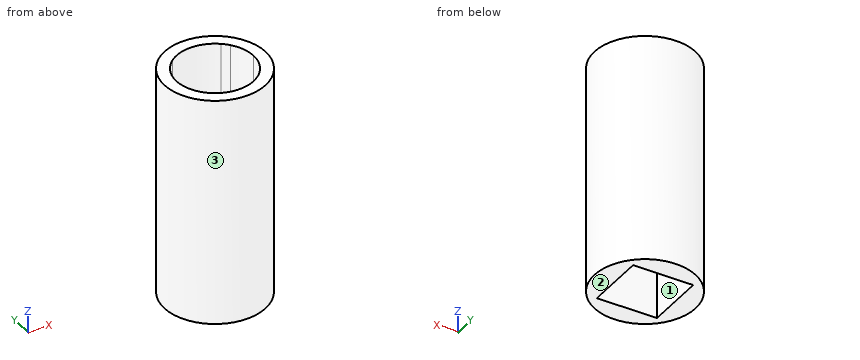
```python
from build123d import *

# Parameters (mm, degrees)
F0_R     = 21
F0_W     = 24.95
F0_H     = 24.95
F1_DEPTH = 45
F2_R     = 21
F3_DEPTH = 50
F4_DEPTH = 5


with BuildPart() as f1:
    # F0 (on Top) → F1 (new body)
    with BuildSketch(Plane.XY):
        Circle(F0_R)
        Rectangle(F0_W, F0_H, mode=Mode.SUBTRACT)
    extrude(amount=F1_DEPTH)

    # F2 (on face) → F3 (join)
    with BuildSketch(Plane.XY.offset(45)):
        Circle(F2_R)
        with BuildLine():
            ThreePointArc((12.475, 10.0585784284), (15.1114608824, 5.3333268229), (16.025, 0))
            ThreePointArc((16.025, 0), (15.1114608824, -5.3333268229), (12.475, -10.0585784284))
            Line((12.475, -10.0585784284), (12.475, -12.475))
            Line((12.475, -12.475), (10.0585784284, -12.475))
            ThreePointArc((10.0585784284, -12.475), (0, -16.025), (-10.0585784284, -12.475))
            Line((-10.0585784284, -12.475), (-12.475, -12.475))
            Line((-12.475, -12.475), (-12.475, -10.0585784284))
            ThreePointArc((-12.475, -10.0585784284), (-16.025, 0), (-12.475, 10.0585784284))
            Line((-12.475, 10.0585784284), (-12.475, 12.475))
            Line((-12.475, 12.475), (-10.0585784284, 12.475))
            ThreePointArc((-10.0585784284, 12.475), (0, 16.025), (10.0585784284, 12.475))
            Line((10.0585784284, 12.475), (12.475, 12.475))
            Line((12.475, 12.475), (12.475, 10.0585784284))
        make_face(mode=Mode.SUBTRACT)
        with BuildLine():
            ThreePointArc((10.0585784284, 12.475), (11.3313861685, 11.3313861685), (12.475, 10.0585784284))
            Line((12.475, 10.0585784284), (12.475, 12.475))
            Line((12.475, 12.475), (10.0585784284, 12.475))
        make_face()
        with BuildLine():
            Line((12.475, -12.475), (12.475, -10.0585784284))
            ThreePointArc((12.475, -10.0585784284), (11.3313861685, -11.3313861685), (10.0585784284, -12.475))
            Line((10.0585784284, -12.475), (12.475, -12.475))
        make_face()
        with BuildLine():
            ThreePointArc((-12.475, 10.0585784284), (-11.3313861685, 11.3313861685), (-10.0585784284, 12.475))
            Line((-10.0585784284, 12.475), (-12.475, 12.475))
            Line((-12.475, 12.475), (-12.475, 10.0585784284))
        make_face()
        with BuildLine():
            Line((-12.475, -12.475), (-10.0585784284, -12.475))
            ThreePointArc((-10.0585784284, -12.475), (-11.3313861685, -11.3313861685), (-12.475, -10.0585784284))
            Line((-12.475, -10.0585784284), (-12.475, -12.475))
        make_face()
    extrude(amount=F3_DEPTH)

    # F2 (on face) → F4 (join)
    with BuildSketch(Plane.XY.offset(45)):
        with BuildLine():
            Line((12.475, -10.0585784284), (12.475, 10.0585784284))
            ThreePointArc((12.475, 10.0585784284), (11.3313861685, 11.3313861685), (10.0585784284, 12.475))
            Line((10.0585784284, 12.475), (-10.0585784284, 12.475))
            ThreePointArc((-10.0585784284, 12.475), (-11.3313861685, 11.3313861685), (-12.475, 10.0585784284))
            Line((-12.475, 10.0585784284), (-12.475, -10.0585784284))
            ThreePointArc((-12.475, -10.0585784284), (-11.3313861685, -11.3313861685), (-10.0585784284, -12.475))
            Line((-10.0585784284, -12.475), (10.0585784284, -12.475))
            ThreePointArc((10.0585784284, -12.475), (11.3313861685, -11.3313861685), (12.475, -10.0585784284))
        make_face()
        with BuildLine():
            ThreePointArc((12.475, -10.0585784284), (15.1114608824, -5.3333268229), (16.025, 0))
            ThreePointArc((16.025, 0), (15.1114608824, 5.3333268229), (12.475, 10.0585784284))
            Line((12.475, 10.0585784284), (12.475, -10.0585784284))
        make_face()
        with BuildLine():
            Line((-12.475, -10.0585784284), (-12.475, 10.0585784284))
            ThreePointArc((-12.475, 10.0585784284), (-16.025, 0), (-12.475, -10.0585784284))
        make_face()
        with BuildLine():
            ThreePointArc((-10.0585784284, -12.475), (0, -16.025), (10.0585784284, -12.475))
            Line((10.0585784284, -12.475), (-10.0585784284, -12.475))
        make_face()
        with BuildLine():
            Line((-10.0585784284, 12.475), (10.0585784284, 12.475))
            ThreePointArc((10.0585784284, 12.475), (0, 16.025), (-10.0585784284, 12.475))
        make_face()
    extrude(amount=F4_DEPTH)


solid = f1.part
```
The listing builds one solid part. Answer for the finished solid, in the listing's coordinates (mm). Face numbers are marked on the shaded views. Coordinates: 2 decimals unless noted, no trailing zeros. Loops run counter-clockwise (first coordinate to the right, second up) from the corner with the lowest first, then second, coordinate; pieces in that order, holes last. Notation, with made-up numbers: (-17, 53.25) -> (-13, 53.25) arc R20 cw to (-13, 74.25) -> close; hole circle Ø2 at (75, 60.25). An arc over 180 degrees is marked (long way). Use one line per item in the form item = value. Start each with the question number.
Item 1: The part is cut by section D-D on z = 38. Determine the outline of the cut face in (x, y) (3 decimals).
Item 2: The part is cut by section B-B on z = 59.5. Determine the outline of the cut face in (x, y) (3 decimals), then the cut area to 3 significant figures.
Item 3: Flat-ended cylindrical pins translate along their axes: pin 1 Ø10 at (x, z) = (-14.5, 77.5) entering from -Y; pin 2 Ø12.5 at (x, z) = (3, 21.5) entering from -Y; pin 3 Ø12.5 at (x, y) = (-5.5, 1) entering from -Z. Find the tip coordinate at first contact, or state that the pin passes through.
Item 4: Consider L1, parallel to Z at x = 8.5, y = -11; L2, parallel to Y at x = -14.5, z = 64.5; L3, parallel to Z at x = 1.5, y = -14. Determine where each line is inside the solid, lowest interval first. Write a range as [from, to].
Item 5: The part is cut by section C-C on y = 3.5. Determine the outline of the cut face in (x, z) (3 decimals), then the cut area to 3 significant figures.
Item 6: The mould has two halves that part along X. Classify the marked faces 1, 2 and 3: released by +X, released by -X, zero draft, split by the parting line, or undercut.
Answer key:
q1.outline = circle Ø42 at (0, 0); hole (-12.475, -12.475) -> (12.475, -12.475) -> (12.475, 12.475) -> (-12.475, 12.475) -> close
q2.outline = circle Ø42 at (0, 0); hole circle Ø32.05 at (0, 0)
q2.area = 579 mm2
q3.pin_1 = -18.73
q3.pin_2 = -21
q3.pin_3 = 45
q4.L1 = [45, 50]
q4.L2 = [-15.19, -6.82], [6.82, 15.19]
q4.L3 = [0, 50]
q5.outline = (-20.706, 0) -> (-12.475, 0) -> (-12.475, 45) -> (12.475, 45) -> (12.475, 0) -> (20.706, 0) -> (20.706, 95) -> (15.638, 95) -> (15.638, 50) -> (-15.638, 50) -> (-15.638, 95) -> (-20.706, 95) -> close
q5.area = 1,400 mm2
q6.face_1 = undercut
q6.face_2 = zero draft
q6.face_3 = split by the parting line
